CAD build for the part. Positions are in the model's coordinates, mm. Round coordinates to 2 decimals unless told otherwise and drop trailing zeros. Order: outer loops, then holes, each group sorted by start corner. A loop starts at its lowest first (then second) coordinate and runs counter-clockwise, first axis right, second up. Notation, with made-up numbers: (-28, -1.5) - (-10, -1.5) arc R26 cw to (-10, 27.5) - close; hole circle Ø4 at (-19.5, 40). An arc over 180 degrees is marked (long way). Write item = value, one per line.
from build123d import *

# Parameters (mm, degrees)
SKETCH1_W           = 114.3
SKETCH1_H           = 101.6
BOSS_EXTRUDE1_DEPTH = 9.525
FILLET1_R           = 3.048
SKETCH3_R           = 2.667
CUT_EXTRUDE1_DEPTH  = 9.525


with BuildPart() as part:
    # Sketch1 → Boss-Extrude1 (new body)
    with BuildSketch(Plane(origin=(0, 0, 0), x_dir=(1, 0, 0), z_dir=(0, 1, 0))):
        Rectangle(SKETCH1_W, SKETCH1_H)
    extrude(amount=BOSS_EXTRUDE1_DEPTH)

    # Fillet1
    fillet1_edges = [part.edges().sort_by_distance(p)[0] for p in [
        (-57.15, 4.7625, -50.8),
        (57.15, 4.7625, -50.8),
        (57.15, 4.7625, 50.8),
        (-57.15, 4.7625, 50.8),
    ]]
    fillet(fillet1_edges, radius=FILLET1_R)

    # Sketch3 → Cut-Extrude1 (cut)
    with BuildSketch(Plane(origin=(0, 9.525, 0), x_dir=(1, 0, 0), z_dir=(0, 1, 0))):
        with Locations((50.8, 44.45)):
            Circle(SKETCH3_R)
        with Locations((25.4, 44.45)):
            Circle(SKETCH3_R)
        with Locations((0, 44.45)):
            Circle(SKETCH3_R)
        with Locations((-25.4, 44.45)):
            Circle(SKETCH3_R)
        with Locations((-50.8, 44.45)):
            Circle(SKETCH3_R)
        with Locations((25.4, -44.45)):
            Circle(SKETCH3_R)
        with Locations((0, -44.45)):
            Circle(SKETCH3_R)
        with Locations((-25.4, -44.45)):
            Circle(SKETCH3_R)
        with Locations((-50.8, -44.45)):
            Circle(SKETCH3_R)
        with Locations((50.8, -44.45)):
            Circle(SKETCH3_R)
        with Locations((38.1, 6.35)):
            Circle(SKETCH3_R)
        with Locations((-38.1, 6.35)):
            Circle(SKETCH3_R)
    extrude(amount=-CUT_EXTRUDE1_DEPTH, mode=Mode.SUBTRACT)


solid = part.part
(1) Band-saw the part on C-C on z = 44.45. List the corners of the cut face in (x, y) (3 decimals), plus the area to 3 significant figures.
Solved:
outline = (-57.15, 0) - (-53.467, 0) - (-53.467, 9.525) - (-57.15, 9.525) - close; (-48.133, 0) - (-28.067, 0) - (-28.067, 9.525) - (-48.133, 9.525) - close; (-22.733, 0) - (-2.667, 0) - (-2.667, 9.525) - (-22.733, 9.525) - close; (2.667, 0) - (22.733, 0) - (22.733, 9.525) - (2.667, 9.525) - close; (28.067, 0) - (48.133, 0) - (48.133, 9.525) - (28.067, 9.525) - close; (53.467, 0) - (57.15, 0) - (57.15, 9.525) - (53.467, 9.525) - close
area = 835 mm²
(2) Probe line 1 along X through (y, z) = (7, 44.45); line 2 along Z through (x, y) = (-25.4, 6.25); line 3 along X through (y, z) = (8, -7). List the from-to ranges inside material, lowest first.
Solved:
line_1 = -57.15 to -53.47, -48.13 to -28.07, -22.73 to -2.67, 2.67 to 22.73, 28.07 to 48.13, 53.47 to 57.15
line_2 = -50.8 to -47.12, -41.78 to 41.78, 47.12 to 50.8
line_3 = -57.15 to -40.69, -35.51 to 35.51, 40.69 to 57.15
(3) Band-saw the part on D-D on y = 5.25. Count the separate pieces of the cut face and the enclosed holes in it, plus the area to 3 significant figures.
Solved:
separate_pieces = 1
enclosed_holes = 12
area = 11,300 mm²
(4) Band-saw the part on B-B on x = -25.4. List the corners of the cut face in (y, z) (3 decimals).
Solved:
outline = (0, -50.8) - (9.525, -50.8) - (9.525, -47.117) - (0, -47.117) - close; (0, -41.783) - (9.525, -41.783) - (9.525, 41.783) - (0, 41.783) - close; (0, 47.117) - (9.525, 47.117) - (9.525, 50.8) - (0, 50.8) - close
(5) Drop flat-ended pins along their axis: pin 1 (7 mm diameter, centred on x = -50.8, z = 44.45, fed in from +Y) (3 decimals); pin 2 (3 mm diameter, centred on x = 0, z = 44.45, fed in from -Y). Give the stop position or say it passes through.
Solved:
pin_1 = 9.525
pin_2 = through
(6) Pull direction Z, two halves, no side cores. Call faces 1 (the cylindrical face through (35.436, 4.829, -6.467)), 2 (the flat face through (-1, 5, 50.8)), 3 (the flat face through (-1, 9.525, -1)): released by +Z, released by -Z, zero draft, split by the parting line, or undercut.
Solved:
face_1 = undercut
face_2 = released by +Z
face_3 = zero draft
(7) Band-saw the part on A-A on z = -6.35. List the corners of the cut face in (x, y) (3 decimals).
Solved:
outline = (-57.15, 0) - (-40.767, 0) - (-40.767, 9.525) - (-57.15, 9.525) - close; (-35.433, 0) - (35.433, 0) - (35.433, 9.525) - (-35.433, 9.525) - close; (40.767, 0) - (57.15, 0) - (57.15, 9.525) - (40.767, 9.525) - close
